Source: CAD feature listing. Evaluate the final solid. Frame: model axes, mm. Face numbers are marked on the shaded views. A direction names the side the tool comes from. Give positions to 0.01 mm unless a question says otherwise; leave off trailing zeros. Write each loop counter-clockwise with the first axis right and the second up, starting at its lowest first coordinate (ties: lowest second). Pieces come first, ordered by that corner, then holes. Notation, with made-up numbers: (81, 51) -> (140, 51) arc R13 ccw to (140, 61) -> close; hole circle Ø5 at (12.25, 86.5). An arc over 180 degrees is marked (long way). Use one line per item in the form item = value. Start each with the question number.
(1) Cut plane B-B, the plane x = 130.5. Output: boundary loops of the cut face in (y, z), and give its area (3 significant figures).
(2) Set-up query: the marked faces 4, 5 and 6. Return all of +Z, -Z, +X, -X, +Y, -Y with unobstructed straight access to the full face (end or side cutting, diameter ignored); none if empty.
(3) Cut plane D-D, the plane z = 26. Count the separate pieces of the cut face and the enclosed holes in it, and give its area (3 significant figures).
(4) Material intervals for line 1 along Y through (x, z) = (84.5, 77); line 2 along Y through (x, z) = (58.5, 26); line 3 along Y through (x, z) = (15, 44.5), sorted ascending. Write a range as from..to.
(5) Cut plane C-C, the plane y = 25. Output: boundary loops of the cut face in (x, z), and give its area (3 significant figures).
(6) First-contact query: P1, Ø3, axis at y = -0.5, z = 50.5, coming from the +X side; P2, Ø1.5, axis at x = 22.5, y = -76.5, coming from the -Z side; P3, Ø1, axis at x = 36.5, y = 37.5, coming from the +Z side; P4, Ø0.8, axis at x = 8, y = -29.5, coming from the -Z side. Flat tips, straight axial feed; report the tip coordinate or a pass-through.
(7) Draft query along X for the marked faces 1, 2 and 3. Return one class per face: pulls with the +X half, pulls with the -X half, needs draft (parallel to the pull), parting line crosses it, or undercut.
(8) Cut plane A-A, the plane z = 84. Output: boundary loops of the cut face in (x, y), and give its area (3 significant figures).
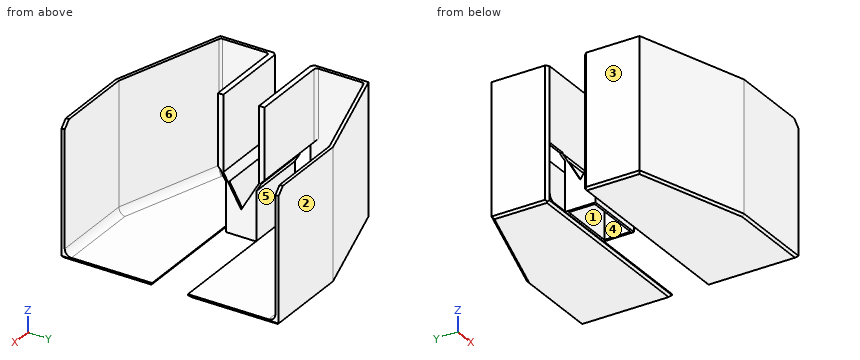
from build123d import *

# Parameters (mm, degrees)
BOSS_EXTRUDE1_DEPTH = 96
BOSS_EXTRUDE2_DEPTH = 2.4
SKETCH3_W           = 2.4
SKETCH3_H           = 61
CUT_EXTRUDE1_DEPTH  = 96
SKETCH4_W           = 143.4
SKETCH4_H           = 41
CUT_EXTRUDE2_DEPTH  = 5
SKETCH9_W           = 83.4
SKETCH9_H           = 55
CUT_EXTRUDE4_DEPTH  = 5
CUT_EXTRUDE3_DEPTH  = 60
BOSS_EXTRUDE3_DEPTH = 45
BOSS_EXTRUDE4_DEPTH = 1.6
CHAMFER1_SIZE       = 5
FILLET1_R           = 2
FILLET3_R           = 5
FILLET4_R           = 2
CHAMFER2_SIZE       = 1.6
CHAMFER3_SIZE       = 2


with BuildPart() as part:
    # Sketch1 → Boss-Extrude1 (new body)
    with BuildSketch(Plane.XY):
        Polygon((145.8, 0), (145.8, 65.8), (82.033733785, 65.8), (0, 40.164458192), (0, 0), (0, -1.6), (145.8, -1.6), align=None)
        Polygon((2.4, 38.4), (2.4, 2.4), (143.4, 2.4), (143.4, 63.4), (82.4, 63.4), align=None, mode=Mode.SUBTRACT)
    extrude(amount=BOSS_EXTRUDE1_DEPTH)

    # Sketch2 → Boss-Extrude2 (add)
    with BuildSketch(Plane(origin=(0, 0, 0), x_dir=(-1, 0, 0), z_dir=(0, 0, -1))):
        Polygon((-145.8, 0), (-145.8, 65.8), (-82.033733785, 65.8), (0, 40.164458192), (0, 0), (0, -1.6), (-145.8, -1.6), align=None)
    extrude(amount=BOSS_EXTRUDE2_DEPTH)

    # Sketch3 → Cut-Extrude1 (cut)
    with BuildSketch(Plane.XY.offset(96)):
        with Locations((144.6, 32.9)):
            Rectangle(SKETCH3_W, SKETCH3_H)
    extrude(amount=-CUT_EXTRUDE1_DEPTH, mode=Mode.SUBTRACT)

    # Sketch4 → Cut-Extrude2 (cut, through all)
    with BuildSketch(Plane(origin=(0, 2.4, 0), x_dir=(1, 0, 0), z_dir=(0, 1, 0))):
        with Locations((74.1, -20.5)):
            Rectangle(SKETCH4_W, SKETCH4_H)
    extrude(amount=-CUT_EXTRUDE2_DEPTH, mode=Mode.SUBTRACT)

    # Sketch9 → Cut-Extrude4 (cut, through all)
    with BuildSketch(Plane(origin=(0, 2.4, 0), x_dir=(1, 0, 0), z_dir=(0, 1, 0))):
        with Locations((104.1, -68.5)):
            Rectangle(SKETCH9_W, SKETCH9_H)
    extrude(amount=-CUT_EXTRUDE4_DEPTH, mode=Mode.SUBTRACT)

    # Sketch5 → Cut-Extrude3 (cut)
    with BuildSketch(Plane(origin=(62.4, 0, 0), x_dir=(0, 0, -1), z_dir=(1, 0, 0))):
        Polygon((-41, 0), (-43.4, 2.4), (-41, 2.4), align=None)
    extrude(amount=-CUT_EXTRUDE3_DEPTH, mode=Mode.SUBTRACT)

    # Sketch6 → Boss-Extrude3 (add)
    with BuildSketch(Plane(origin=(62.4, 0, 0), x_dir=(0, 0, -1), z_dir=(1, 0, 0))):
        Polygon((-40.2, 0), (-41, 0), (-41, -1.6), (-40.2, -1.6), (-33.964617093, -5.2), (2.4, -5.2), (2.4, -3.6), (-33.964617093, -3.6), align=None)
    extrude(amount=-BOSS_EXTRUDE3_DEPTH)

    # Sketch8 → Boss-Extrude4 (add)
    with BuildSketch(Plane(origin=(62.4, 0, 0), x_dir=(0, 0, -1), z_dir=(1, 0, 0))):
        Polygon((-33.964617093, -5.2), (2.4, -26.195121467), (2.4, -5.2), align=None)
    boss_extrude4 = extrude(amount=-BOSS_EXTRUDE4_DEPTH)

    # Mirror1: Boss-Extrude4 across plane
    add(boss_extrude4.mirror(Plane(origin=(39.9, 0, 0), x_dir=(0, 0, 1), z_dir=(1, 0, 0))))

    # Chamfer1
    chamfer1_edges = [part.edges().sort_by_distance(p)[0] for p in [
        (145.8, 64.6, 96),
    ]]
    chamfer(chamfer1_edges, length=CHAMFER1_SIZE)

    # Fillet1
    fillet1_edges = [part.edges().sort_by_distance(p)[0] for p in [
        (2.4, 2.4, 69.7),
    ]]
    fillet(fillet1_edges, radius=FILLET1_R)

    # Fillet3
    fillet3_edges = [part.edges().sort_by_distance(p)[0] for p in [
        (42.4, 50.9, 0),
        (2.4, 18.4, 0),
        (114.1, 63.4, 0),
    ]]
    fillet(fillet3_edges, radius=FILLET3_R)

    # Fillet4
    fillet4_edges = [part.edges().sort_by_distance(p)[0] for p in [
        (2.4, 38.4, 50.5),
    ]]
    fillet(fillet4_edges, radius=FILLET4_R)

    # Chamfer2
    chamfer2_edges = [part.edges().sort_by_distance(p)[0] for p in [
        (145.8, 32.1, -2.4),
        (72.9, -1.6, -2.4),
        (0, 19.282229096, -2.4),
        (41.016866893, 52.982229096, -2.4),
        (113.916866893, 65.8, -2.4),
    ]]
    chamfer(chamfer2_edges, length=CHAMFER2_SIZE)

    # Chamfer3
    chamfer3_edges = [part.edges().sort_by_distance(p)[0] for p in [
        (0, -1.6, 47.6),
    ]]
    chamfer(chamfer3_edges, length=CHAMFER3_SIZE)

    # Mirror2: part across plane


with BuildPart() as part_1:
    add(part.part)
    add(part.part.mirror(Plane.ZX.offset(-14.897560734)))


solid = part_1.part
Geometry says:
q1.outline = (-95.6, -0.8) -> (-94, -2.4) -> (-29.8, -2.4) -> (-28.2, -0.8) -> (-28.2, 0) -> (-88.2, 0) arc R5 cw to (-93.2, 5) -> (-93.2, 96) -> (-95.6, 96) -> close; (-1.6, -0.8) -> (0, -2.4) -> (64.2, -2.4) -> (65.8, -0.8) -> (65.8, 96) -> (63.4, 96) -> (63.4, 5) arc R5 cw to (58.4, 0) -> (-1.6, 0) -> close
q1.area = 790 mm^2
q2.face_4 = +Z, -Z
q2.face_5 = -Z, +X, -X
q2.face_6 = +Z, +X
q3.separate_pieces = 4
q3.enclosed_holes = 0
q3.area = 1,080 mm^2
q4.line_1 = -95.6..-93.2, 63.4..65.8
q4.line_2 = -88.24..-85.73, -26.2..-24.6, -5.2..-3.6, 55.93..58.45
q4.line_3 = -74.65..-72.13, -32.2..-28.2, -1.6..2.4, 42.34..44.85
q5.outline = (0, -0.8) -> (1.6, -2.4) -> (144.2, -2.4) -> (145.8, -0.8) -> (145.8, 0) -> (7.4, 0) arc R5 cw to (2.4, 5) -> (2.4, 96) -> (0, 96) -> close
q5.area = 583 mm^2
q6.P1 = 62.4
q6.P2 = -2.02
q6.P3 = 0
q6.P4 = -2.4
q7.face_1 = undercut
q7.face_2 = needs draft
q7.face_3 = pulls with the -X half
q8.outline = (0, -69.96) -> (82.03, -95.6) -> (145.8, -95.6) -> (145.8, -93.2) -> (82.4, -93.2) -> (3.8, -68.63) arc R2 cw to (2.4, -66.72) -> (2.4, -34.2) arc R2 cw to (4.4, -32.2) -> (62.4, -32.2) -> (62.4, -28.2) -> (2, -28.2) -> (0, -30.2) -> close; (0, 0.4) -> (2, -1.6) -> (62.4, -1.6) -> (62.4, 2.4) -> (4.4, 2.4) arc R2 cw to (2.4, 4.4) -> (2.4, 36.93) arc R2 cw to (3.8, 38.84) -> (82.4, 63.4) -> (145.8, 63.4) -> (145.8, 65.8) -> (82.03, 65.8) -> (0, 40.16) -> close
q8.area = 1,390 mm^2
